The model under review builds one solid part; all positions refer to its coordinate system, in mm. Round coordinates to 2 decimals unless told otherwise and drop trailing zeros. Write each loop counter-clockwise with the first axis right and the second up, starting at its lowest first coordinate (ties: lowest second). Pieces come first, ordered by that corner, then holes. Notation, with made-up numbers: (-12, 52.25) -> (8, 52.25) arc R27 ccw to (8, 85.25) -> close; hole circle Ø11 at (-28.75, 15.25). An arc over 180 degrees is marked (long way). Return JSON: item names as keys, results as strings. Group by question number.
1. Take a section at B-B, the plane x = -34.5. Write out the cut boundary in (y, z), then the cut area to 3 significant figures.
2. Take a section at A-A, the plane z = -22. Write out the cut boundary in (x, y).
3. For line 1 along X through (y, z) = (2.85, -122); line 2 along Z through (x, y) = (-29, 3.3); line 3 along Z through (x, y) = (42.5, 2.9), list the stretches that pass through material, from the lowest coordinate up. Write a range as from..to.
4. Clearance check with a flat-ended pin moving along its axis: P1, Ø4, axis at x = 74.5, z = -140, coming from the +Y side. State where the tip first meets the part, or that it passes through.
from build123d import *

# Parameters (mm, degrees)
CROQUIS1_W              = 167
CROQUIS1_H              = 340
CROQUIS1_R              = 2.6
SALIENTE_EXTRUIR1_DEPTH = 5
SKETCH1_W               = 127
SKETCH1_H               = 300
CUT_EXTRUDE1_DEPTH      = 10


with BuildPart() as part:
    # Croquis1 → Saliente-Extruir1 (new body)
    with BuildSketch(Plane(origin=(0, 0, 0), x_dir=(1, 0, 0), z_dir=(0, 1, 0))):
        Rectangle(CROQUIS1_W, CROQUIS1_H)
        with Locations(Location((-74.5, 140, 0), (0, 0, 270))):
            Circle(CROQUIS1_R, mode=Mode.SUBTRACT)
        with Locations(Location((-74.5, 0, 0), (0, 0, 270))):
            Circle(CROQUIS1_R, mode=Mode.SUBTRACT)
        with Locations(Location((-74.5, -140, 0), (0, 0, 270))):
            Circle(CROQUIS1_R, mode=Mode.SUBTRACT)
        with Locations(Location((74.5, 140, 0), (0, 0, 270))):
            Circle(CROQUIS1_R, mode=Mode.SUBTRACT)
        with Locations(Location((74.5, -140, 0), (0, 0, 270))):
            Circle(CROQUIS1_R, mode=Mode.SUBTRACT)
        with Locations(Location((74.5, 0, 0), (0, 0, 270))):
            Circle(CROQUIS1_R, mode=Mode.SUBTRACT)
        with Locations(Location((-43.5, 160, 0), (0, 0, 270))):
            Circle(CROQUIS1_R, mode=Mode.SUBTRACT)
        with Locations(Location((43.5, 160, 0), (0, 0, 270))):
            Circle(CROQUIS1_R, mode=Mode.SUBTRACT)
        with Locations(Location((-43.5, -160, 0), (0, 0, 270))):
            Circle(CROQUIS1_R, mode=Mode.SUBTRACT)
        with Locations(Location((43.5, -160, 0), (0, 0, 270))):
            Circle(CROQUIS1_R, mode=Mode.SUBTRACT)
    extrude(amount=SALIENTE_EXTRUIR1_DEPTH)

    # Sketch1 → Cut-Extrude1 (cut)
    with BuildSketch(Plane(origin=(0, 5, 0), x_dir=(1, 0, 0), z_dir=(0, 1, 0))):
        Rectangle(SKETCH1_W, SKETCH1_H)
    extrude(amount=-CUT_EXTRUDE1_DEPTH, mode=Mode.SUBTRACT)


solid = part.part
Output:
{
 "1": {"outline": "(0, -170) -> (5, -170) -> (5, -150) -> (0, -150) -> close; (0, 150) -> (5, 150) -> (5, 170) -> (0, 170) -> close", "area": "200 mm^2"},
 "2": {"outline": "(-83.5, 0) -> (-63.5, 0) -> (-63.5, 5) -> (-83.5, 5) -> close; (63.5, 0) -> (83.5, 0) -> (83.5, 5) -> (63.5, 5) -> close"},
 "3": {"line 1": "x = -83.5..-63.5, 63.5..83.5", "line 2": "z = -170..-150, 150..170", "line 3": "z = -170..-162.4, -157.6..-150, 150..157.6, 162.4..170"},
 "4": {"P1": "passes through"}
}
